Check sheet for the modelled part. Datum: model origin and axes. Units: mm. Give positions to 0.01 mm unless a question says otherwise; leave off trailing zeros. Order: outer loops, then holes, each group sorted by start corner. A loop starts at its lowest first (then second) coordinate and runs counter-clockwise, first axis right, second up. Notation, with made-up numbers: (-16.75, -22.75) - (21.25, -22.75) arc R19 cw to (21.25, -2.75) - close; hole circle Ø8 at (27.5, 34.25). An arc over 180 degrees is marked (long way). Answer in a Markdown table with one row per item.
from build123d import *

# Parameters (mm, degrees)
SKETCH_1_R          = 85.5
SKETCH_1_R_2        = 2.65
EXTRUDE_1_DEPTH     = 2
SKETCH_2_W          = 40
SKETCH_2_H          = 100
CUT_EXTRUDE_2_DEPTH = 2
SKETCH_4_R          = 2.65
CUT_EXTRUDE_3_DEPTH = 2
SKETCH_5_W          = 100
SKETCH_5_H          = 100
CUT_EXTRUDE_4_DEPTH = 2


with BuildPart() as part:
    # 草图1 → 凸台-拉伸1 (new body)
    with BuildSketch(Plane(origin=(0, 0, 0), x_dir=(1, 0, 0), z_dir=(0, 1, 0))):
        with Locations(Location((0, 0, 0), (0, 0, 270))):
            Circle(SKETCH_1_R)
        with Locations(Location((0, 79, 0), (0, 0, 270))):
            Circle(SKETCH_1_R_2, mode=Mode.SUBTRACT)
        with Locations(Location((79, 0, 0), (0, 0, 270))):
            Circle(SKETCH_1_R_2, mode=Mode.SUBTRACT)
        with Locations(Location((0, -79, 0), (0, 0, 270))):
            Circle(SKETCH_1_R_2, mode=Mode.SUBTRACT)
        with Locations(Location((-79, 0, 0), (0, 0, 270))):
            Circle(SKETCH_1_R_2, mode=Mode.SUBTRACT)
    extrude(amount=EXTRUDE_1_DEPTH)

    # 草图2 → 切除-拉伸2 (cut)
    with BuildSketch(Plane(origin=(0, 2, 0), x_dir=(1, 0, 0), z_dir=(0, 1, 0))):
        with Locations((-20, 0)):
            Rectangle(SKETCH_2_W, SKETCH_2_H)
        with Locations((20, 0)):
            Rectangle(SKETCH_2_W, SKETCH_2_H)
    extrude(amount=-CUT_EXTRUDE_2_DEPTH, mode=Mode.SUBTRACT)

    # 草图4 → 切除-拉伸3 (cut)
    with BuildSketch(Plane(origin=(0, 2, 0), x_dir=(1, 0, 0), z_dir=(0, 1, 0))):
        with Locations(Location((0, 64.031242374, 0), (0, 0, 270))):
            Circle(SKETCH_4_R)
        with Locations(Location((64.031242374, 0, 0), (0, 0, 270))):
            Circle(SKETCH_4_R)
        with Locations(Location((0, -64.031242374, 0), (0, 0, 270))):
            Circle(SKETCH_4_R)
        with Locations(Location((-64.031242374, 0, 0), (0, 0, 270))):
            Circle(SKETCH_4_R)
    extrude(amount=-CUT_EXTRUDE_3_DEPTH, mode=Mode.SUBTRACT)

    # 草图5 → 切除-拉伸4 (cut)
    with BuildSketch(Plane(origin=(0, 2, 0), x_dir=(1, 0, 0), z_dir=(0, 1, 0))):
        Rectangle(SKETCH_5_W, SKETCH_5_H)
    extrude(amount=-CUT_EXTRUDE_4_DEPTH, mode=Mode.SUBTRACT)


solid = part.part
(1) Mould release check, pull along Z, two halves, no side actions. Record for faces 1 (the flat face through (1, 2, 56)), 2 (the cylindrical face through (84.772, 0.986, -11.13)), 3 (the cylindrical face through (0.796, 1.014, 66.559)), 4 (the cylindrical face through (-61.4, 1, -0.3)): pulls with the +Z half, pulls with the -Z half, needs draft (parallel to the pull), parting line crosses it, or undercut.
Geometry says:
| item | result |
|---|---|
| face 1 | needs draft |
| face 2 | parting line crosses it |
| face 3 | undercut |
| face 4 | undercut |
(2) Cross-section at D-D, the plane z = -64.5. Record the cut outline in (x, y).
Geometry says:
| item | result |
|---|---|
| outline | (-56.12, 0) - (-2.61, 0) - (-2.61, 2) - (-56.12, 2) - close; (2.61, 0) - (56.12, 0) - (56.12, 2) - (2.61, 2) - close |
(3) Cross-section at C-C, the plane y = 1.45. Give the number of separate pieces and of enclosed holes in the cut face, then the cut area to 3 significant figures.
Geometry says:
| item | result |
|---|---|
| separate pieces | 1 |
| enclosed holes | 9 |
| area | 12,800 mm² |
(4) Cross-section at B-B, the plane z = 0. Record the cut outline in (x, y), then the cut area to 3 significant figures.
Geometry says:
| item | result |
|---|---|
| outline | (-85.5, 0) - (-81.65, 0) - (-81.65, 2) - (-85.5, 2) - close; (-76.35, 0) - (-66.68, 0) - (-66.68, 2) - (-76.35, 2) - close; (-61.38, 0) - (-50, 0) - (-50, 2) - (-61.38, 2) - close; (50, 0) - (61.38, 0) - (61.38, 2) - (50, 2) - close; (66.68, 0) - (76.35, 0) - (76.35, 2) - (66.68, 2) - close; (81.65, 0) - (85.5, 0) - (85.5, 2) - (81.65, 2) - close |
| area | 99.6 mm² |
(5) Cross-section at A-A, the plane x = 0. Record the cut outline in (y, z), then the cut area to 3 significant figures.
Geometry says:
| item | result |
|---|---|
| outline | (0, -85.5) - (2, -85.5) - (2, -81.65) - (0, -81.65) - close; (0, -76.35) - (2, -76.35) - (2, -66.68) - (0, -66.68) - close; (0, -61.38) - (2, -61.38) - (2, -50) - (0, -50) - close; (0, 50) - (2, 50) - (2, 61.38) - (0, 61.38) - close; (0, 66.68) - (2, 66.68) - (2, 76.35) - (0, 76.35) - close; (0, 81.65) - (2, 81.65) - (2, 85.5) - (0, 85.5) - close |
| area | 99.6 mm² |
(6) Gauge pin test, flat ends, axial feed: P1, Ø3, axis at x = -64.03, z = 0, coming from the -Y side; P2, Ø1, axis at x = 58, y = 1.5, coming from the -Z side; P3, Ø1, axis at y = 0.5, z = 10.5, coming from the -X side; P4, Ø1, axis at x = -5, y = 1, coming from the -Z side. Record the tip position at first contact, or that the pin passes through.
Geometry says:
| item | result |
|---|---|
| P1 | through |
| P2 | z = -63.28 |
| P3 | x = -84.91 |
| P4 | z = -85.38 |
(7) Thickness scan on L1, parallel to X at y = 0.5, z = 0; L2, parallel to X at y = 0.7, z = 22.5; L3, parallel to X at y = 1.35, z = -17.5. Record the ranges inside material, lowest first.
Geometry says:
| item | result |
|---|---|
| L1 | -85.5 to -81.65, -76.35 to -66.68, -61.38 to -50, 50 to 61.38, 66.68 to 76.35, 81.65 to 85.5 |
| L2 | -82.49 to -50, 50 to 82.49 |
| L3 | -83.69 to -50, 50 to 83.69 |
